The model under review builds one solid part; all positions refer to its coordinate system, in mm. Round coordinates to 2 decimals unless told otherwise and drop trailing zeros. Loops run counter-clockwise (first coordinate to the right, second up) from the corner with the lowest first, then second, coordinate; pieces in that order, holes last. Notation, with made-up numbers: M 60,87 L 83,87 A23 ccw 83,119 Z; hole C 27.5,68.25 d11. An arc over 180 degrees is marked long. Return JSON: item names as keys, results as strings. Group by question number.
Q1. Consider section D-D (z = -150.5). State the section outline as (x, y) points.
Q2. To check wall thickness, follow line 1 along Y through (x, z) = (1.75, -270); line 2 along Y through (x, z) = (2.1, -60.5); line 3 along Z through (x, y) = (1.15, 165.5). State the ranges of each line that lie inside material, in increasing order.
Q3. Consider section B-B (y = 160). State the section outline as (x, z) points, and give its area (3 significant figures).
Q4. Consider section A-A (z = -270). State the section outline as (x, y) points, and give its area (3 significant figures).
Q5. Clearance check with flat-ended pins moving along their axes: pin 1 Ø1 at (x, z) = (0.5, -309.5) entering from -Y; pin 2 Ø1.5 at (x, z) = (0.5, -239.5) entering from +Y; pin 3 Ø1.5 at (x, y) = (2, 531) entering from +Z. State where each tip first meets the part, or that it passes through.
Q6. Consider section C-C (x = 2.3). State the section outline as (y, z) points.
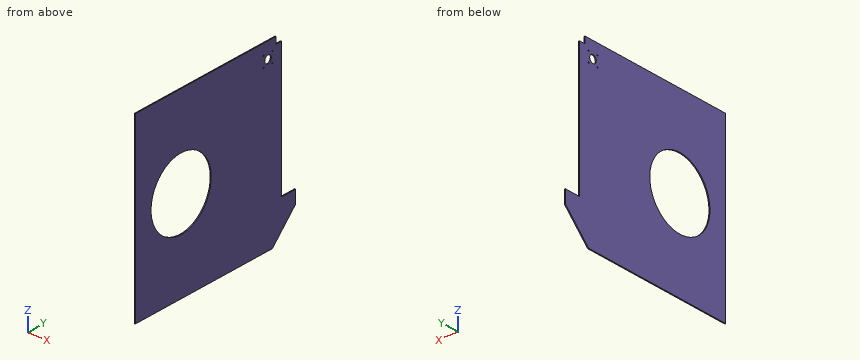
from build123d import *

# Parameters (mm, degrees)
BOSS_EXTRUDE1_DEPTH = 3
SKETCH3_R           = 105
CUT_EXTRUDE1_DEPTH  = 3
SKETCH4_R           = 1.75
SKETCH4_R_2         = 11.5
CUT_EXTRUDE2_DEPTH  = 15


with BuildPart() as part:
    # Sketch1 → Boss-Extrude1 (new body)
    with BuildSketch(Plane(origin=(0, 0, 0), x_dir=(0, 0, -1), z_dir=(1, 0, 0))):
        Polygon((540, 475.629480553), (540, 478.284271247), (458.284271247, 560), (420, 560), (420, 510), (20, 510), (20, 491.519731167), (0, 491.519731167), (0, 475.629480553), (0, 0), (540, 0), align=None)
    extrude(amount=BOSS_EXTRUDE1_DEPTH)

    # Sketch3 → Cut-Extrude1 (cut)
    with BuildSketch(Plane.ZY):
        with Locations((-270, 160)):
            Circle(SKETCH3_R)
    extrude(amount=-CUT_EXTRUDE1_DEPTH, mode=Mode.SUBTRACT)

    # Sketch4 → Cut-Extrude2 (cut)
    with BuildSketch(Plane(origin=(3, 0, 0), x_dir=(0, 0, -1), z_dir=(1, 0, 0))):
        with Locations((32.367626301, 478.88695563)):
            Circle(SKETCH4_R)
        with Locations((32.367626301, 447.88695563)):
            Circle(SKETCH4_R)
        with Locations((63.367626301, 447.88695563)):
            Circle(SKETCH4_R)
        with Locations((63.367626301, 478.88695563)):
            Circle(SKETCH4_R)
        with Locations((47.867626301, 463.38695563)):
            Circle(SKETCH4_R_2)
    extrude(amount=-CUT_EXTRUDE2_DEPTH, mode=Mode.SUBTRACT)


solid = part.part
Values:
{
 "1": {"outline": "M 0,0 L 3,0 L 3,510 L 0,510 Z"},
 "2": {"line 1": "y = 0 to 55, 265 to 510", "line 2": "y = 0 to 510", "line 3": "z = -540 to -374.86, -165.14 to 0"},
 "3": {"outline": "M 0,-540 L 3,-540 L 3,-375 L 0,-375 Z; M 0,-165 L 3,-165 L 3,0 L 0,0 Z", "area": "990 mm2"},
 "4": {"outline": "M 0,0 L 3,0 L 3,55 L 0,55 Z; M 0,265 L 3,265 L 3,510 L 0,510 Z", "area": "900 mm2"},
 "5": {"pin 1": "stops at y = 0", "pin 2": "stops at y = 510", "pin 3": "stops at z = -420"},
 "6": {"outline": "M 0,-540 L 478.28,-540 L 560,-458.28 L 560,-420 L 510,-420 L 510,-20 L 491.52,-20 L 491.52,0 L 0,0 Z; hole C 160,-270 d210; hole C 447.89,-63.37 d3.5; hole C 447.89,-32.37 d3.5; hole C 463.39,-47.87 d23; hole C 478.89,-63.37 d3.5; hole C 478.89,-32.37 d3.5"}
}
